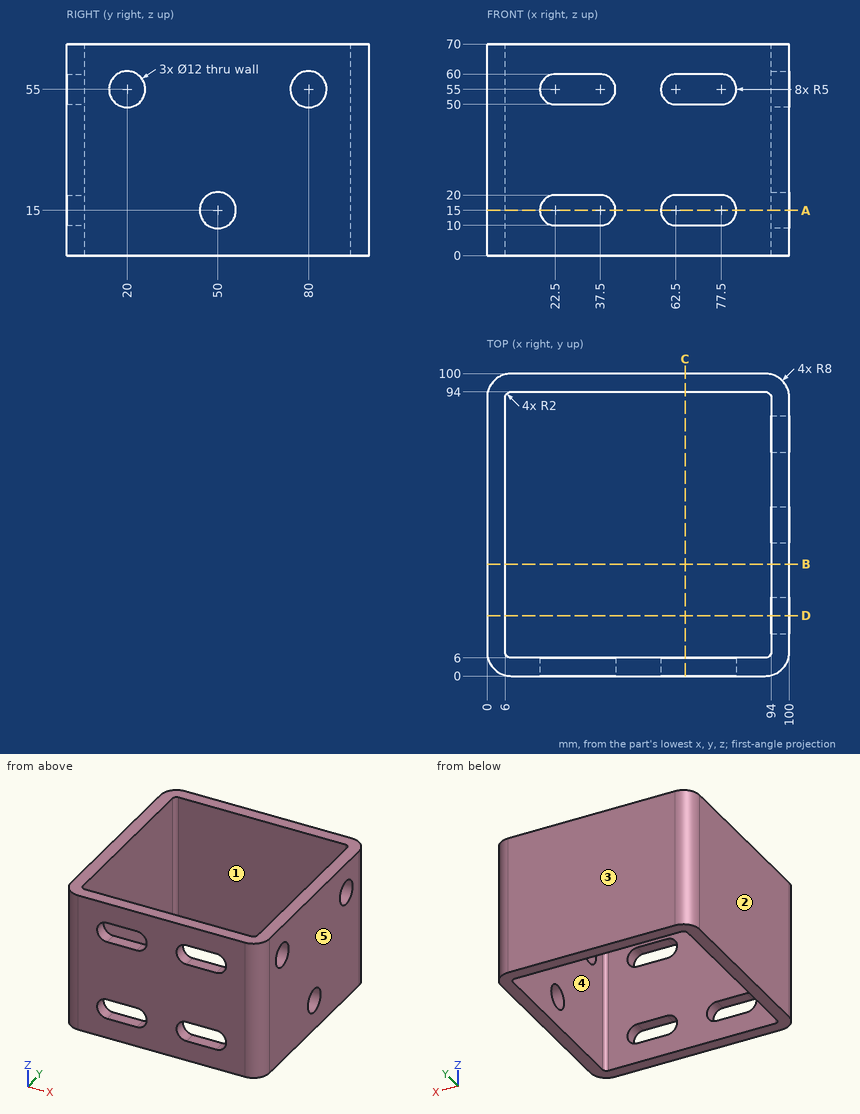
Could you check a few things on this drawing? It's one solid part, dimensions in mm from its lowest x, y, z. A direction names the side the tool comes from. Give positions to 0.01 mm unless a question says otherwise; leave off trailing zeros. Write each loop counter-clockwise with the first axis right and the second up, starting at its lowest first coordinate (ties: lowest second). Pieces come first, ordered by that corner, then holes. Notation, with made-up numbers: (17.5, 35) -> (42.5, 35) arc R20 cw to (42.5, 64) -> close; hole circle Ø6 at (-9.5, -36). An arc over 180 degrees is marked (long way). Answer as CSV lines item,"result". Start each with the question number.
(1) If we section it at C-C, the plane x = 65.5: Write out the boundary of the cut face in (y, z), and give its area (3 significant figures).
(2) Which directions (+Z, -Z, +X, -X, +Y, -Y) give clear straight access to the entire face, cutting with the end or side of a thin tool? Please do the marked faces 4 and 5.
(3) Please list where these lines run through material, in increasing order: line 1 (X direction, y = 61, z = 15.5); line 2 (Y direction, x = 98, z = 55).
(4) If we mould it in two halves opening along Y, with no side actions, what happens to the marked faces 1, 2 and 3? For each: +Y half, -Y half, draft (parallel to the pull), parting line (faces both ways), or undercut.
(5) If we section it at A-A, the plane z = 15: Write out the boundary of the cut face in (x, y).
(6) If we section it at B-B, the plane y = 37: Write out the boundary of the cut face in (x, z), and give its area (3 significant figures).
(7) If we section it at D-D, the plane y = 20: Write out the boundary of the cut face in (x, z), and give its area (3 significant figures).
(8) I'm going to push a flat-ended pin straight in: pin 1 Ø7 at (y, z) = (80, 55) entering from +X. Where does the tip first touch, or does it pass through?
Answer list:
1,outline,"(0, 0) -> (6, 0) -> (6, 10) -> (0, 10) -> close; (0, 20) -> (6, 20) -> (6, 50) -> (0, 50) -> close; (0, 60) -> (6, 60) -> (6, 70) -> (0, 70) -> close; (94, 0) -> (100, 0) -> (100, 70) -> (94, 70) -> close"
1,area,"720 mm^2"
2,face 4,"+Z, -Z"
2,face 5,"+Z, -Z, +X, +Y, -Y"
3,line 1,"0 to 6, 94 to 100"
3,line 2,"2.71 to 14, 26 to 74, 86 to 97.29"
4,face 1,"undercut"
4,face 2,"draft"
4,face 3,"+Y half"
5,outline,"(0, 8) arc R8 ccw to (8, 0) -> (17.5, 0) -> (17.5, 6) -> (8, 6) arc R2 cw to (6, 8) -> (6, 92) arc R2 cw to (8, 94) -> (92, 94) arc R2 cw to (94, 92) -> (94, 56) -> (100, 56) -> (100, 92) arc R8 ccw to (92, 100) -> (8, 100) arc R8 ccw to (0, 92) -> close; (42.5, 0) -> (57.5, 0) -> (57.5, 6) -> (42.5, 6) -> close; (82.5, 0) -> (92, 0) arc R8 ccw to (100, 8) -> (100, 44) -> (94, 44) -> (94, 8) arc R2 cw to (92, 6) -> (82.5, 6) -> close"
6,outline,"(0, 0) -> (6, 0) -> (6, 70) -> (0, 70) -> close; (94, 0) -> (100, 0) -> (100, 70) -> (94, 70) -> close"
6,area,"840 mm^2"
7,outline,"(0, 0) -> (6, 0) -> (6, 70) -> (0, 70) -> close; (94, 0) -> (100, 0) -> (100, 49) -> (94, 49) -> close; (94, 61) -> (100, 61) -> (100, 70) -> (94, 70) -> close"
7,area,"768 mm^2"
8,pin 1,"x = 6"
